Part model, mm, in its own coordinate system. Face numbers are marked on the shaded views. Round coordinates to 2 decimals unless told otherwise and drop trailing zeros. Loops run counter-clockwise (first coordinate to the right, second up) from the corner with the lowest first, then second, coordinate; pieces in that order, holes last. Notation, with made-up numbers: M -30.75,-34.5 L -3.75,-34.5 A22 cw -3.75,-26.5 Z; hole C 36,-38 d10. An arc over 180 degrees is marked long. Answer as CSV lines item,"result". Start each with the question number.
Item 1: Wall check: line 1 (Z direction, x = 0, y = -9.5); line 2 (Z direction, x = 3, y = -7.75); line 3 (X direction, y = -1, z = 82.5). Give the ranges that are in metal, low to high.
Item 2: Mould opens along X. For the marked faces 1, 2 and 3 say: pulls with the +X half, pulls with the -X half, needs draft (parallel to the pull), parting line crosses it, or undercut.
Item 3: Band-saw the part on B-B (x = 0). Give the cut face in (y, z).
Item 4: Band-saw the part on C-C (y = -8). Give the cut face in (x, z), and give its area (3 significant figures).
Item 5: Drop flat-ended pins along their axis: pin 1 Ø2 at (x, y) = (5, -2.5) entering from -Z; pin 2 Ø4 at (x, y) = (1.5, -7.5) entering from +Z. Give the stop position or say it passes through.
Item 6: Band-saw the part on A-A (z = 75). Give the cut face in (x, y).
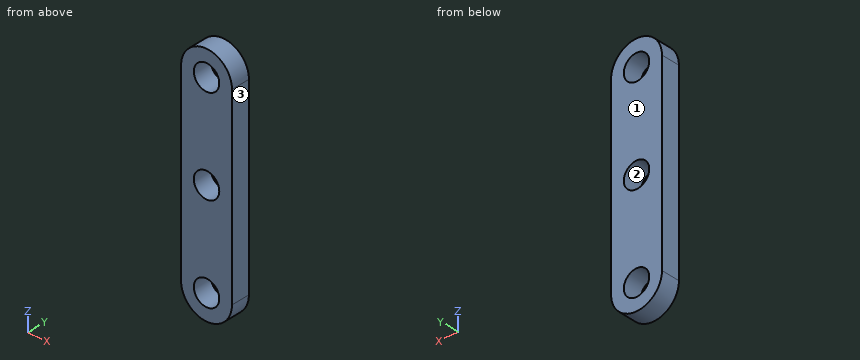
```python
from build123d import *

# Parameters (mm, degrees)
F1_DEPTH = 15
F2_R     = 10
F3_DEPTH = 25
F4_R     = 10
F5_DEPTH = 25


with BuildPart() as f1:
    # F0 (on Front) → F1 (new body)
    with BuildSketch(Plane.XZ):
        with BuildLine():
            ThreePointArc((-20, 0), (0, -20), (20, 0))
            ThreePointArc((20, 0), (0, 20), (-20, 0))
        make_face()
        with BuildLine():
            ThreePointArc((-20, 0), (0, 20), (20, 0))
            Line((20, 0), (20, 150))
            ThreePointArc((20, 150), (0, 130), (-20, 150))
            Line((-20, 150), (-20, 0))
        make_face()
        with BuildLine():
            ThreePointArc((-20, 150), (0, 130), (20, 150))
            ThreePointArc((20, 150), (0, 170), (-20, 150))
        make_face()
    extrude(amount=F1_DEPTH)

    # F2 (on face) → F3 (cut)
    with BuildSketch(Plane.XZ.offset(15)):
        with Locations((0, 150)):
            Circle(F2_R)
        Circle(F2_R)
    extrude(amount=-F3_DEPTH, mode=Mode.SUBTRACT)

    # F4 (on face) → F5 (cut)
    with BuildSketch(Plane.XZ.offset(15)):
        with Locations((0, 75)):
            Circle(F4_R)
    extrude(amount=-F5_DEPTH, mode=Mode.SUBTRACT)


solid = f1.part
```
Answer block:
1,line 1,"z = -20 to -10, 10 to 65, 85 to 140, 160 to 170"
1,line 2,"z = -19.77 to -9.54, 9.54 to 65.46, 84.54 to 140.46, 159.54 to 169.77"
1,line 3,"x = -20 to -6.61, 6.61 to 20"
2,face 1,"needs draft"
2,face 2,"undercut"
2,face 3,"pulls with the +X half"
3,outline,"M -15,-20 L 0,-20 L 0,-10 L -15,-10 Z; M -15,10 L 0,10 L 0,65 L -15,65 Z; M -15,85 L 0,85 L 0,140 L -15,140 Z; M -15,160 L 0,160 L 0,170 L -15,170 Z"
4,outline,"M -20,0 A20 ccw 20,0 L 20,150 A20 ccw -20,150 Z; hole C 0,0 d20; hole C 0,75 d20; hole C 0,150 d20"
4,area,"6,310 mm^2"
5,pin 1,"stops at z = -19.6"
5,pin 2,"stops at z = 170"
6,outline,"M -20,-15 L -10,-15 L -10,0 L -20,0 Z; M 10,-15 L 20,-15 L 20,0 L 10,0 Z"
